Source: CAD feature listing. Evaluate the final solid. Frame: model axes, mm. A direction names the side the tool comes from. Give positions to 0.01 mm unless a question says otherwise; leave off trailing zeros. Write each loop counter-clockwise with the first axis right and the second up, starting at its lowest first coordinate (ties: lowest second). Pieces come first, ordered by that corner, then holes. Notation, with made-up numbers: (45.25, -28.75) -> (93.25, -28.75) arc R23 ccw to (93.25, 5.25) -> close; hole circle Ø4 at (15.25, -3.5). An arc over 180 degrees is marked (long way). Write item = value, one per line.
from build123d import *

# Parameters (mm, degrees)
SKETCH1_R           = 3
BOSS_EXTRUDE1_DEPTH = 3
CHAMFER1_SIZE       = 0.3
CUT_EXTRUDE1_DEPTH  = 2.5
CHAMFER2_SIZE       = 0.3
SKETCH3_R           = 1.5
BOSS_EXTRUDE2_DEPTH = 30
CHAMFER3_SIZE       = 0.2


with BuildPart() as part:
    # Sketch1 → Boss-Extrude1 (new body)
    with BuildSketch(Plane(origin=(0, 0, 0), x_dir=(1, 0, 0), z_dir=(0, 1, 0))):
        with Locations(Location((0, 0, 0), (0, 0, 270))):  # turned: the seam where the file's is
            Circle(SKETCH1_R)
    extrude(amount=BOSS_EXTRUDE1_DEPTH)

    # Chamfer1
    chamfer1_edges = [part.edges().sort_by_distance(p)[0] for p in [
        (0, 3, -3),
    ]]
    chamfer(chamfer1_edges, length=CHAMFER1_SIZE)

    # Sketch2 → Cut-Extrude1 (cut)
    with BuildSketch(Plane(origin=(0, 3, 0), x_dir=(1, 0, 0), z_dir=(0, 1, 0))):
        Polygon((1.732050808, 0), (0.866025404, 1.5), (-0.866025404, 1.5), (-1.732050808, 0), (-0.866025404, -1.5), (0.866025404, -1.5), align=None)
    extrude(amount=-CUT_EXTRUDE1_DEPTH, mode=Mode.SUBTRACT)

    # Chamfer2
    chamfer2_edges = [part.edges().sort_by_distance(p)[0] for p in [
        (1.299038106, 3, 0.75),
        (1.299038106, 3, -0.75),
        (0, 3, -1.5),
        (-1.299038106, 3, -0.75),
        (-1.299038106, 3, 0.75),
        (0, 3, 1.5),
    ]]
    chamfer(chamfer2_edges, length=CHAMFER2_SIZE)

    # Sketch3 → Boss-Extrude2 (add)
    with BuildSketch(Plane.XZ):
        with Locations(Location((0, 0, 0), (0, 0, 90))):  # turned: the seam where the file's is
            Circle(SKETCH3_R)
    extrude(amount=BOSS_EXTRUDE2_DEPTH)

    # Chamfer3
    chamfer3_edges = [part.edges().sort_by_distance(p)[0] for p in [
        (0, -30, -1.5),
    ]]
    chamfer(chamfer3_edges, length=CHAMFER3_SIZE)


solid = part.part
1) Cut plane A-A (y = 1). Return the cut outline in (x, z), then the cut area to 3 significant figures.
Computed:
outline = circle Ø6 at (0, 0); hole (-1.73, 0) -> (-0.87, -1.5) -> (0.87, -1.5) -> (1.73, 0) -> (0.87, 1.5) -> (-0.87, 1.5) -> close
area = 20.5 mm²
2) Draft query along Z for faces 1 (the flat face through (-1.42, 2.85, -0.84)), 2 (the cylindrical face through (0.9, 1.33, 2.86)), 3 (the flat face through (-2, 3, -1)). Return one class per face: pulls with the +Z half, pulls with the -Z half, needs draft (parallel to the pull), parting line crosses it, or undercut.
Computed:
face_1 = undercut
face_2 = parting line crosses it
face_3 = needs draft
3) Cut plane B-B (x = 0). Return the cut outline in (y, z), then the cut area to 3 significant figures.
Computed:
outline = (-30, -1.3) -> (-29.8, -1.5) -> (0, -1.5) -> (0, -3) -> (2.7, -3) -> (3, -2.7) -> (3, -1.8) -> (2.7, -1.5) -> (0.5, -1.5) -> (0.5, 1.5) -> (2.7, 1.5) -> (3, 1.8) -> (3, 2.7) -> (2.7, 3) -> (0, 3) -> (0, 1.5) -> (-29.8, 1.5) -> (-30, 1.3) -> close
area = 100 mm²
4) Access query for faces 4 (the flat face through (0, -30, 0)), 5 (the cylindrical face through (-0.45, -14.69, 1.43)), 6 (the flat face through (-1.305, 1.615, 0.74)). Directions: +Z, -Z, +X, -X, +Y, -Y. A direction counts if a zero-diameter tool reaches every point of the face in a straight line with its end or side. Return the directions, or none.
Computed:
face_4 = +Z, -Z, +X, -X, -Y
face_5 = -Y
face_6 = +Y
5) Contact query for flat-ended pins moving along their axis: pin 1 (1 mm diameter, centred on x = 0, y = -21, fed in from +Z); pin 2 (2.5 mm diameter, centred on x = 0, z = 0, fed in from +Y). Output: stop coordinate, or through.
Computed:
pin_1 = 1.5
pin_2 = 0.5
6) Material intervals for L1, parallel to Y at x = -0.65, z = 1.9; L2, parallel to X at y = -21, z = 0.05; L3, parallel to X at y = -10, z = -0.55, sorted ascending.
Computed:
L1 = 0 to 3
L2 = -1.5 to 1.5
L3 = -1.4 to 1.4
